Geometry: final body of the model. Coordinates: model frame, mm. A direction names the side the tool comes from. Round coordinates to 2 decimals unless told otherwise and drop trailing zeros. Loops run counter-clockwise (first coordinate to the right, second up) from the corner with the lowest first, then second, coordinate; pieces in that order, holes last. Notation, with made-up numbers: (54.25, 61) -> (86.25, 61) arc R21 ccw to (86.25, 66) -> close; hole circle Ø7 at (-36, 64.25). An arc over 180 degrees is marked (long way). Answer in a Markdown table with one row per item.
```python
from build123d import *

# Parameters (mm, degrees)
SKIZZE1_W                       = 16
SKIZZE1_H                       = 15
AUFSATZ_LINEAR_AUSTRAGEN1_DEPTH = 10
SCHNITT_LINEAR_AUSTRAGEN1_DEPTH = 5
SCHNITT_LINEAR_AUSTRAGEN2_DEPTH = 6


with BuildPart() as part:
    # Skizze1 → Aufsatz-Linear austragen1 (new body)
    with BuildSketch(Plane.XY):
        with Locations((8, 7.5)):
            Rectangle(SKIZZE1_W, SKIZZE1_H)
    extrude(amount=AUFSATZ_LINEAR_AUSTRAGEN1_DEPTH)

    # Skizze2 → Schnitt-Linear austragen1 (cut)
    with BuildSketch(Plane.XY.offset(10)):
        with BuildLine():
            Line((0, 12.5), (7, 12.5))
            ThreePointArc((7, 12.5), (12, 7.5), (7, 2.5))
            Line((7, 2.5), (0, 2.5))
            ThreePointArc((0, 2.5), (-5, 7.5), (0, 12.5))
        make_face()
    extrude(amount=-SCHNITT_LINEAR_AUSTRAGEN1_DEPTH, mode=Mode.SUBTRACT)

    # Skizze3 → Schnitt-Linear austragen2 (cut, through all)
    with BuildSketch(Plane.XY.offset(5)):
        with BuildLine():
            Line((0, 9.75), (7, 9.75))
            ThreePointArc((7, 9.75), (9.25, 7.5), (7, 5.25))
            Line((7, 5.25), (0, 5.25))
            ThreePointArc((0, 5.25), (-2.25, 7.5), (0, 9.75))
        make_face()
    extrude(amount=-SCHNITT_LINEAR_AUSTRAGEN2_DEPTH, mode=Mode.SUBTRACT)


solid = part.part
```
Item 1: Reachability of faces 1 (the face through (8, 0, 5)), 2 (the face through (4, 5.25, 3)), 3 (the face through (4, 2.5, 8)) from +Z, -Z, +X, -X, +Y, -Y: full face, straight path, thin tool, end or side. Return the list, or none.
Answer:
| item | result |
|---|---|
| face 1 | +Z, -Z, +X, -X, -Y |
| face 2 | +Z, -Z, -X |
| face 3 | +Z, -X |
Item 2: Cut plane D-D (y = 7.5). Output: boundary loops of the cut face in (x, z).
Answer:
| item | result |
|---|---|
| outline | (9.25, 0) -> (16, 0) -> (16, 10) -> (12, 10) -> (12, 5) -> (9.25, 5) -> close |
Item 3: Cut plane C-C (x = 9.5). Output: boundary loops of the cut face in (y, z).
Answer:
| item | result |
|---|---|
| outline | (0, 0) -> (15, 0) -> (15, 10) -> (11.83, 10) -> (11.83, 5) -> (3.17, 5) -> (3.17, 10) -> (0, 10) -> close |
Item 4: Line query: probe 1 along Y at (x, z) = (6.75, 5.5); probe 2 along Y at (x, z) = (1.5, 1.25); probe 3 along Z at (x, y) = (8.25, 11.75). Output: solid intervals per line, ascending. Write a range as [from, to].
Answer:
| item | result |
|---|---|
| probe 1 | y = [0, 2.5], [12.5, 15] |
| probe 2 | y = [0, 5.25], [9.75, 15] |
| probe 3 | z = [0, 5] |
Item 5: Draft query along Y for faces 4 (the face through (8, 15, 5)), 5 (the face through (0, 2, 4)), 6 (the face through (3, 9.75, 3)). Return one class per face: pulls with the +Y half, pulls with the -Y half, needs draft (parallel to the pull), parting line crosses it, or undercut.
Answer:
| item | result |
|---|---|
| face 4 | pulls with the +Y half |
| face 5 | needs draft |
| face 6 | undercut |
Item 6: Pin query (flat end, axial travel): pin 1 Ø6 at (x, y) = (2, 8.5) entering from +Z. Return the tip coordinate at first contact, or that it passes through.
Answer:
| item | result |
|---|---|
| pin 1 | stops at z = 5 |
Item 7: Cut plane A-A (x = 6.25). Output: boundary loops of the cut face in (y, z).
Answer:
| item | result |
|---|---|
| outline | (0, 0) -> (5.25, 0) -> (5.25, 5) -> (2.5, 5) -> (2.5, 10) -> (0, 10) -> close; (9.75, 0) -> (15, 0) -> (15, 10) -> (12.5, 10) -> (12.5, 5) -> (9.75, 5) -> close |
Item 8: Cut plane B-B (z = 5.5). Output: boundary loops of the cut face in (x, y).
Answer:
| item | result |
|---|---|
| outline | (0, 0) -> (16, 0) -> (16, 15) -> (0, 15) -> (0, 12.5) -> (7, 12.5) arc R5 cw to (7, 2.5) -> (0, 2.5) -> close |
